Build history of the part. All positions in model axes, mm. A direction names the side the tool comes from. Give positions to 0.01 mm unless a question says otherwise; leave off trailing zeros. Order: outer loops, then holes, each group sorted by start corner. A loop starts at its lowest first (then second) coordinate and runs counter-clockwise, first axis right, second up. Notation, with made-up numbers: (-34, -1) - (12, -1) arc R24 cw to (12, 11) - close; hole circle Ø8 at (-14, 24.25). An arc over 180 degrees is marked (long way). Answer in a Markdown table with one row per item.
```python
from build123d import *

# Parameters (mm, degrees)
SKETCH_1_R          = 4.5
EXTRUDE_2_DEPTH     = 4
CUT_EXTRUDE_1_DEPTH = 83.559069762
FILLET_1_R          = 3
SKETCH_6_R          = 1.7
CUT_EXTRUDE_2_DEPTH = 83.559069762


with BuildPart() as part:
    # 草图1 → 凸台-拉伸2 (new body)
    with BuildSketch(Plane.XY):
        with BuildLine():
            Line((20, -60), (20, 60))
            ThreePointArc((20, 60), (0, 80), (-20, 60))
            Line((-20, 60), (-20, -60))
            ThreePointArc((-20, -60), (0, -80), (20, -60))
        make_face()
        with Locations((0, 60)):
            Circle(SKETCH_1_R, mode=Mode.SUBTRACT)
        with Locations((0, -60)):
            Circle(SKETCH_1_R, mode=Mode.SUBTRACT)
    extrude(amount=EXTRUDE_2_DEPTH)

    # 草图4 → 切除-拉伸1 (cut, through all)
    with BuildSketch(Plane.XY.offset(4)):
        Polygon((-14, -18.844505579), (11.137802231, 44), (-14, 44), align=None)
        Polygon((14, -44), (14, 18.844505579), (-11.137802231, -44), align=None)
    extrude(amount=-CUT_EXTRUDE_1_DEPTH, mode=Mode.SUBTRACT)

    # 圆角1
    fillet_1_edges = [part.edges().sort_by_distance(p)[0] for p in [
        (14, -44, 2),
        (-11.137802231, -44, 2),
        (14, 18.844505579, 2),
        (-14, -18.844505579, 2),
        (-14, 44, 2),
        (11.137802231, 44, 2),
    ]]
    fillet(fillet_1_edges, radius=FILLET_1_R)

    # 草图6 → 切除-拉伸2 (cut, through all)
    with BuildSketch(Plane.XY.offset(4)):
        with Locations((0, 50)):
            Circle(SKETCH_6_R)
        with Locations((-8.660254038, 55)):
            Circle(SKETCH_6_R)
        with Locations((-8.660254038, 65)):
            Circle(SKETCH_6_R)
        with Locations((0, 70)):
            Circle(SKETCH_6_R)
        with Locations((8.660254038, 65)):
            Circle(SKETCH_6_R)
        with Locations((8.660254038, 55)):
            Circle(SKETCH_6_R)
        with Locations(Location((0, -70, 0), (0, 0, 180))):
            Circle(SKETCH_6_R)
        with Locations(Location((-8.660254038, -65, 0), (0, 0, 180))):
            Circle(SKETCH_6_R)
        with Locations(Location((-8.660254038, -55, 0), (0, 0, 180))):
            Circle(SKETCH_6_R)
        with Locations(Location((0, -50, 0), (0, 0, 180))):
            Circle(SKETCH_6_R)
        with Locations(Location((8.660254038, -55, 0), (0, 0, 180))):
            Circle(SKETCH_6_R)
        with Locations(Location((8.660254038, -65, 0), (0, 0, 180))):
            Circle(SKETCH_6_R)
    extrude(amount=-CUT_EXTRUDE_2_DEPTH, mode=Mode.SUBTRACT)


solid = part.part
```
1. Two-plate mould, pull along Y, no slides. Class faces 1 (the face through (-10.28, -65.51, 2.03)), 2 (the face through (-20, 1, 2)), 3 (the face through (0, 80, 2)): +Y half, -Y half, draft (parallel to the pull), parting line (faces both ways), or undercut.
Check result:
| item | result |
|---|---|
| face 1 | undercut |
| face 2 | draft |
| face 3 | +Y half |
2. Cut at A-A on y = -50. Write the cut outline in (x, z).
Check result:
| item | result |
|---|---|
| outline | (-20, 0) - (-1.7, 0) - (-1.7, 4) - (-20, 4) - close; (1.7, 0) - (20, 0) - (20, 4) - (1.7, 4) - close |
3. Cut at B-B on z = 1.15. Count the separate pieces of the cut face and the enclosed holes in it, and give its area (3 significant figures).
Check result:
| item | result |
|---|---|
| separate pieces | 1 |
| enclosed holes | 16 |
| area | 4,320 mm² |
4. Which spindle directions (+Z, -Z, +X, -X, +Y, -Y) get a long thin tool onto all of the face, cutting with end or side? Do faces 4 (the face through (-13.1, 43.14, 1.97)), 5 (the face through (0, 1, 0)). Say none if no direction does.
Check result:
| item | result |
|---|---|
| face 4 | +Z, -Z |
| face 5 | -Z, +X, -X, +Y, -Y |
5. Drop a flat-ended pin along its axis: P1, Ø2, axis at x = 8.66, y = -55, coming from the +Z side. Give the stop position or say it passes through.
Check result:
| item | result |
|---|---|
| P1 | passes through |
6. Probe line 1 (X direction, y = -55, z = 1.9); line 2 (X direction, y = -65.5, z = 2.6); line 3 (Y direction, x = -10, z = 0.2). List the from-to ranges inside material, lowest first.
Check result:
| item | result |
|---|---|
| line 1 | x = -20 to -10.36, -6.96 to 6.96, 10.36 to 20 |
| line 2 | x = -19.23 to -10.29, -7.04 to 7.04, 10.29 to 19.23 |
| line 3 | y = -77.32 to -66.05, -63.95 to -56.05, -53.95 to -6.1, 44 to 53.95, 56.05 to 63.95, 66.05 to 77.32 |
7. Cut at D-D on x = -16.5. Write the cut outline in (y, z), and give its area (3 significant figures).
Check result:
| item | result |
|---|---|
| outline | (-71.3, 0) - (71.3, 0) - (71.3, 4) - (-71.3, 4) - close |
| area | 570 mm² |
8. Cut at C-C on y = 70. Write the cut outline in (x, z), and give its area (3 significant figures).
Check result:
| item | result |
|---|---|
| outline | (-17.32, 0) - (-1.7, 0) - (-1.7, 4) - (-17.32, 4) - close; (1.7, 0) - (17.32, 0) - (17.32, 4) - (1.7, 4) - close |
| area | 125 mm² |
